Design review of the part built by this model. Coordinates are the model's own, in mm. A direction names the side the tool comes from. Round coordinates to 2 decimals unless told otherwise and drop trailing zeros. Order: outer loops, then holes, each group sorted by start corner. A loop starts at its lowest first (then second) coordinate and runs counter-clockwise, first axis right, second up. Notation, with made-up numbers: M 67.25,69.5 L 116.25,69.5 A22 cw 116.25,90.5 Z; hole C 19,87 d1. An arc over 180 degrees is marked long. Use a Markdown table: item, result. Add a question column.
(1) Take a section at A-A (y = -23.25). Write out the cut boundary in (x, z), then the cut area to 3 significant figures.
(2) For pin 1 (6 mm diameter, centred on y = -17.5, z = 25, fed in from -X); pin 2 (1 mm diameter, centred on x = -1.5, y = -9, fed in from -Z); pin 3 (5 mm diameter, centred on x = -2, y = -11, fed in from -Z), all flat-tipped, find the tip position at first contact; note any pin that passes through.
(3) Take a section at D-D (z = 15.5). Write out the cut boundary in (x, y).
(4) Take a section at B-B (z = 27). Write out the cut boundary in (x, y), then the cut area to 3 significant figures.
(5) Take a section at C-C (x = -8). Write out the cut boundary in (y, z).
(6) To check wall thickness, follow probe 1 along X at (y, z) = (-3.5, 22); probe 2 along Z at (x, y) = (16, -16.5); probe 3 along Z at (x, y) = (11, -11). State the ranges of each line that lie inside material, in increasing order. Write a range as from..to.
(7) Machinability: for faces 1 (the face through (0, -13, 16)), 2 (the face through (12.7, -13, 17)), 3 (the face through (7, -13, 44.45)), which of the approach directions +Z, -Z, +X, -X, +Y, -Y give a long, thin tool a straight path to every point of the face, cutting with its end or side? Answer none if there is none.
```python
from build123d import *

# Parameters (mm, degrees)
F1_DEPTH = 25.4
F3_DEPTH = 25.4
F5_DEPTH = 12.7
F7_DEPTH = 12.7


with BuildPart() as f1:
    # F0 (on Front) → F1 (new body)
    with BuildSketch(Plane.XZ):
        Polygon((-12.7, 25.4), (0, 25.4), (0, 0), (12.7, 0), (12.7, 25.4), (25.4, 25.4), (25.4, 44.45), (-12.7, 44.45), align=None)
    extrude(amount=F1_DEPTH)

    # F2 (on face) → F3 (cut)
    with BuildSketch(Plane(origin=(0, 0, 0), x_dir=(0, -1, 0), z_dir=(-1, 0, 0))):
        Polygon((25.4, 9.339999), (0, 0), (25.4, 0), align=None)
    extrude(amount=-F3_DEPTH, mode=Mode.SUBTRACT)

    # F4 (on face) → F5 (cut)
    with BuildSketch(Plane(origin=(-12.7, 0, 0), x_dir=(0, -1, 0), z_dir=(-1, 0, 0))):
        Polygon((25.4, 25.4), (25.4, 32.345079), (0, 25.4), align=None)
    extrude(amount=-F5_DEPTH, mode=Mode.SUBTRACT)

    # F6 (on face) → F7 (cut)
    with BuildSketch(Plane.YZ.offset(25.4)):
        Polygon((-25.4, 25.4), (0, 25.4), (-25.4, 34.925), align=None)
    extrude(amount=-F7_DEPTH, mode=Mode.SUBTRACT)


solid = f1.part
```
Verdict:
| question | item | result |
|---|---|---|
| 1 | outline | M -12.7,31.76 L 0,31.76 L 0,8.55 L 12.7,8.55 L 12.7,34.12 L 25.4,34.12 L 25.4,44.45 L -12.7,44.45 Z |
| 1 | area | 748 mm^2 |
| 2 | pin 1 | stops at x = 0 |
| 2 | pin 2 | stops at z = 27.72 |
| 2 | pin 3 | stops at z = 3.49 |
| 3 | outline | M 0,-25.4 L 12.7,-25.4 L 12.7,0 L 0,0 Z |
| 4 | outline | M -12.7,-5.85 L 0,-5.85 L 0,-25.4 L 12.7,-25.4 L 12.7,-4.27 L 25.4,-4.27 L 25.4,0 L -12.7,0 Z |
| 4 | area | 451 mm^2 |
| 5 | outline | M -25.4,32.35 L 0,25.4 L 0,44.45 L -25.4,44.45 Z |
| 6 | probe 1 | x = 0..12.7 |
| 6 | probe 2 | z = 31.59..44.45 |
| 6 | probe 3 | z = 4.04..44.45 |
| 7 | face 1 | -Z, -X, -Y |
| 7 | face 2 | -Z, +X, -Y |
| 7 | face 3 | +Z, +X, -X, +Y, -Y |
